Input: part model. Units: mm. Frame: model coordinates. A direction names the side the tool comes from. Round coordinates to 2 decimals unless told otherwise and drop trailing zeros. Loops run counter-clockwise (first coordinate to the right, second up) from the corner with the lowest first, then second, coordinate; pieces in that order, holes last. Notation, with made-up numbers: M 16,-34 L 66,-34 A32 cw 66,-2 Z; hole C 51,0 d8. An arc over 180 degrees is marked long. Return JSON: item names as keys, results as strings. Group by question number.
1) Material intervals for line 1 (X direction, y = -2, z = 0.6); line 2 (X direction, y = 30, z = 2.2); line 3 (Y direction, x = -29, z = 2.35), sorted ascending. Write a range as from..to.
2) Section A-A (y = -3). Output: boundary loops of the cut face in (x, z), plus the area to 3 significant figures.
3) Contact query for flat-ended pins moving along their axis: P1, Ø0.9, axis at y = -19, z = 1.5, coming from the +X side; P2, Ø0.9, axis at x = -39, z = 1.5, coming from the -Y side; P3, Ø6, axis at x = -6.26, y = -1.57, coming from the +Z side; P4, Ø0.9, axis at y = 27, z = 1.5, coming from the +X side. Output: stop coordinate, or through.
4) Access query for faces 1 (the face through (-39, 11.466, 1)), 2 (the face through (-32, -17.565, 1)), 3 (the face through (50, 1.789, 1)), 4 (the face through (50, -7.888, 1)), 5 (the face through (51.453, 16, 1)). Directions: +Z, -Z, +X, -X, +Y, -Y. A direction counts if a zero-diameter tool reaches every point of the face in a straight line with its end or side. Return the directions, or none.
5) Mould query, pull axis Y, two halves, no side actions, for faces 6 (the face through (-39, -7.888, 1)), 7 (the face through (-39, 21.143, 1)), 8 (the face through (-0.782, -19, 1)), 9 (the face through (-39, 1.789, 1)). Classes: +Y half, -Y half, draft (parallel to the pull), parting line (faces both ways), or undercut.
6) Section D-D (x = 38.5). Output: boundary loops of the cut face in (y, z).
7) Section C-C (z = 2.45). Count the separate pieces of the cut face and the enclosed holes in it, plus the area to 3 significant figures.
8) Section B-B (x = 10). Output: boundary loops of the cut face in (y, z), plus the area to 3 significant figures.
from build123d import *

# Parameters (mm, degrees)
BOSS_EXTRUDE1_DEPTH = 3
SKETCH2_R           = 3.841087015
CUT_EXTRUDE1_DEPTH  = 3


with BuildPart() as part:
    # Sketch1 → Boss-Extrude1 (new body)
    with BuildSketch(Plane.XY):
        Polygon((-37.70901952, -17.564925379), (-25.400175445, -17.564925379), (-25.400175445, -20.564925379), (-13.09133137, -20.564925379), (-13.09133137, -17.564925379), (-0.782487296, -17.564925379), (-0.782487296, -20.564925379), (11.526356779, -20.564925379), (11.526356779, -17.564925379), (23.835200854, -17.564925379), (23.835200854, -20.564925379), (36.144044929, -20.564925379), (36.144044929, -17.564925379), (48.500170095, -17.564925379), (48.500170095, -7.888062048), (51.452889003, -7.888062048), (51.452889003, 1.788801284), (48.452889003, 1.788801284), (48.452889003, 11.465664615), (51.452889003, 11.465664615), (51.452889003, 21.142527947), (48.452889003, 21.142527947), (48.452889003, 30.819391278), (51.452889003, 30.819391278), (51.452889003, 40.49625461), (48.452889003, 40.49625461), (48.452889003, 50.173117941), (-37.70901952, 50.173117941), (-37.70901952, 40.49625461), (-40.70901952, 40.49625461), (-40.70901952, 30.819391278), (-37.70901952, 30.819391278), (-37.70901952, 21.142527947), (-40.70901952, 21.142527947), (-40.70901952, 11.465664615), (-37.70901952, 11.465664615), (-37.70901952, 1.788801284), (-40.70901952, 1.788801284), (-40.70901952, -7.888062048), (-37.70901952, -7.888062048), align=None)
    extrude(amount=BOSS_EXTRUDE1_DEPTH)

    # Sketch2 → Cut-Extrude1 (cut)
    with BuildSketch(Plane.XY.offset(3)):
        with Locations((-6.25812843, -1.568095487)):
            Circle(SKETCH2_R)
        with Locations((11.456834914, -1.568095487)):
            Circle(SKETCH2_R)
    extrude(amount=-CUT_EXTRUDE1_DEPTH, mode=Mode.SUBTRACT)


solid = part.part
Returned:
{
 "1": {"line 1": "x = -40.71..-10.07, -2.44..7.64, 15.27..51.45", "line 2": "x = -37.71..48.45", "line 3": "y = -17.56..50.17"},
 "2": {"outline": "M -40.71,0 L -9.82,0 L -9.82,3 L -40.71,3 Z; M -2.69,0 L 7.89,0 L 7.89,3 L -2.69,3 Z; M 15.02,0 L 51.45,0 L 51.45,3 L 15.02,3 Z", "area": "234 mm^2"},
 "3": {"P1": "stops at x = 36.14", "P2": "stops at y = -7.89", "P3": "passes through", "P4": "stops at x = 48.45"},
 "4": {"face 1": "+Z, -Z, -X", "face 2": "+Z, -Z, -X, -Y", "face 3": "+Z, -Z, +X", "face 4": "+Z, -Z, +X, -Y", "face 5": "+Z, -Z, +X, +Y, -Y"},
 "5": {"face 6": "-Y half", "face 7": "undercut", "face 8": "draft", "face 9": "undercut"},
 "6": {"outline": "M -17.56,0 L 50.17,0 L 50.17,3 L -17.56,3 Z"},
 "7": {"separate pieces": "1", "enclosed holes": "2", "area": "6,030 mm^2"},
 "8": {"outline": "M -20.56,0 L -5.12,0 L -5.12,3 L -20.56,3 Z; M 1.99,0 L 50.17,0 L 50.17,3 L 1.99,3 Z", "area": "191 mm^2"}
}
